Design review of the part built by this model. Coordinates are the model's own, in mm. Face numbers are marked on the shaded views. A direction names the side the tool comes from. Round coordinates to 2 decimals unless told otherwise and drop trailing zeros. Loops run counter-clockwise (first coordinate to the right, second up) from the corner with the lowest first, then second, coordinate; pieces in that order, holes last. Notation, with made-up numbers: (66.5, 10) - (115.5, 10) arc R17 cw to (115.5, 33) - close; hole circle Ø10 at (-20, -9.75). An arc over 180 degrees is marked (long way). Return JSON: item names as keys, results as strings. Group by question number.
(1) Clearance check with flat-ended pins moving along their axes: pin 1 (9 mm diameter, centred on x = 7.62, z = -6.35, fed in from +Y); pin 2 (12 mm diameter, centred on x = 401.5, y = 127, fed in from +Z). State where each tip first meets the part, or that it passes through.
(2) We need section C-C, the plane y = 35.5. Write out the cut boundary in (x, z).
(3) We need section A-A, the plane x = 336. Write out the cut boundary in (y, z).
(4) Wall thickness on L1, parallel to X at y = -0.1, z = -6.35; L2, parallel to Z at x = 390.5, y = 69; L3, parallel to Y at x = 128.5, z = -9: over which ranges is each line inside the solid? List them lowest first. Write a range as [from, to].
(5) For the marked faces 1 and 2, list the 3-axis set-ups (+Z, -Z, +X, -X, +Y, -Y) from which the entire face can be reached by the end or side of a thin tool; tool diameter is ignored.
(6) We need section D-D, the plane x = 228.6. Write out the cut boundary in (y, z), and give its area (3 significant figures).
(7) We need section B-B, the plane z = -14.5. Write out the cut boundary in (x, y).
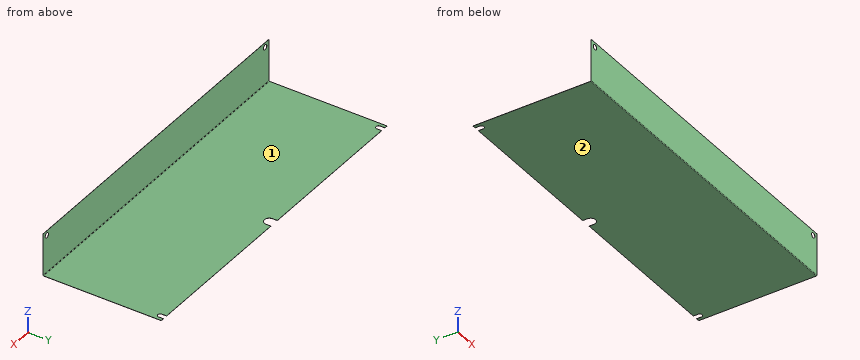
from build123d import *

# Parameters (mm, degrees)
SKETCH1_W                    = 457.2
SKETCH1_H                    = 57.15
BASE_FLANGE1_DEPTH           = 0.15875
EDGE_FLANGE1_STRIP_W         = 2.1082
EDGE_FLANGE1_STRIP_H         = 0.15875
EDGE_FLANGE1_STRIP_CUT_DEPTH = 457.2
EDGE_FLANGE1_DEPTH           = 457.2
CUT_EXTRUDE1_DEPTH           = 488.3392299
F_1_4_CLEARANCE_HOLE2_D      = 6.7564
F_1_4_CLEARANCE_HOLE2_DEPTH  = 25.4
F_1_4_CLEARANCE_HOLE2_TIP    = 2.029827343


# Sheet-metal steps are written as plain solids
with BuildPart() as part:
    # Sketch1 → Base-Flange1 (new body)
    with BuildSketch(Plane(origin=(0, 0, 0), x_dir=(1, 0, 0), z_dir=(0, 1, 0))):
        with Locations((228.6, 28.575)):
            Rectangle(SKETCH1_W, SKETCH1_H)
    extrude(amount=-BASE_FLANGE1_DEPTH)

    # Edge-Flange1 strip (across the edge) → Edge-Flange1 strip cut (cut)
    with BuildSketch(Plane(origin=(457.2, 0, -57.15), x_dir=(0, 0, 1), z_dir=(-1, 0, 0))):
        with Locations((-0.15875, -0.079375)):
            Rectangle(EDGE_FLANGE1_STRIP_W, EDGE_FLANGE1_STRIP_H)
    extrude(amount=EDGE_FLANGE1_STRIP_CUT_DEPTH, mode=Mode.SUBTRACT)

    # Edge-Flange1 section (across the edge) → Edge-Flange1 (add)
    with BuildSketch(Plane(origin=(457.2, 0, -57.15), x_dir=(0, 0, 1), z_dir=(-1, 0, 0))):
        with BuildLine():
            Line((0, 0.7366), (0, 158.75))
            Line((0, 158.75), (0.15875, 158.75))
            Line((0.15875, 158.75), (0.15875, 0.7366))
            ThreePointArc((0.15875, 0.7366), (0.374495145, 0.215745145), (0.89535, 0))
            Line((0.89535, 0), (0.89535, -0.15875))
            ThreePointArc((0.89535, -0.15875), (0.262241943, 0.103491943), (0, 0.7366))
        make_face()
    extrude(amount=EDGE_FLANGE1_DEPTH)

    # Sketch9 → Cut-Extrude1 (cut, through all)
    with BuildSketch(Plane(origin=(0, 0, -57.15), x_dir=(-1, 0, 0), z_dir=(0, 0, -1))):
        with BuildLine():
            Line((-446.278, 152.4), (-446.278, 158.75))
            Line((-446.278, 158.75), (-452.882, 158.75))
            Line((-452.882, 158.75), (-452.882, 152.4))
            ThreePointArc((-452.882, 152.4), (-449.58, 149.098), (-446.278, 152.4))
        make_face()
        with BuildLine():
            Line((-10.922, 152.4), (-10.922, 158.75))
            Line((-10.922, 158.75), (-4.318, 158.75))
            Line((-4.318, 158.75), (-4.318, 152.4))
            ThreePointArc((-4.318, 152.4), (-7.62, 149.098), (-10.922, 152.4))
        make_face()
        with BuildLine():
            Line((-235.204, 152.4), (-235.204, 158.75))
            Line((-235.204, 158.75), (-221.996, 158.75))
            Line((-221.996, 158.75), (-221.996, 152.4))
            ThreePointArc((-221.996, 152.4), (-228.6, 145.796), (-235.204, 152.4))
        make_face()
    extrude(amount=-CUT_EXTRUDE1_DEPTH, mode=Mode.SUBTRACT)

    # 1/4 Clearance Hole2
    with Locations(Plane(origin=(7.62, -0.15875, -6.35), x_dir=(0, 0, -1), z_dir=(0, -1, 0))):
        with Locations((0, 0), (0, 441.96)):
            Hole(F_1_4_CLEARANCE_HOLE2_D / 2, depth=F_1_4_CLEARANCE_HOLE2_DEPTH)
            with Locations((0, 0, -(F_1_4_CLEARANCE_HOLE2_DEPTH + F_1_4_CLEARANCE_HOLE2_TIP / 2))):  # 118° drill point
                Cone(0, F_1_4_CLEARANCE_HOLE2_D / 2, F_1_4_CLEARANCE_HOLE2_TIP, mode=Mode.SUBTRACT)


solid = part.part
Solutions:
{
 "1": {"pin 1": "y = 0", "pin 2": "z = -56.99"},
 "2": {"outline": "(0, -57.15) - (457.2, -57.15) - (457.2, -56.99) - (0, -56.99) - close"},
 "3": {"outline": "(-0.16, -56.25) arc R0.9 ccw to (0.74, -57.15) - (158.75, -57.15) - (158.75, -56.99) - (0.74, -56.99) arc R0.74 cw to (0, -56.25) - (0, 0) - (-0.16, 0) - close"},
 "4": {"L1": "[0, 4.24], [11, 446.2], [452.96, 457.2]", "L2": "[-57.15, -56.99]", "L3": "[-0.16, 0]"},
 "5": {"face 1": "+Z, +X, -X, +Y", "face 2": "-Z, +X, -X, +Y, -Y"},
 "6": {"outline": "(-0.16, -56.25) arc R0.9 ccw to (0.74, -57.15) - (145.8, -57.15) - (145.8, -56.99) - (0.74, -56.99) arc R0.74 cw to (0, -56.25) - (0, 0) - (-0.16, 0) - close", "area": "32.2 mm^2"},
 "7": {"outline": "(0, -0.16) - (457.2, -0.16) - (457.2, 0) - (0, 0) - close"}
}
